The figure shows three views and two pictorial views of one solid part (mm, origin at its lowest corner). Answer the questions. Round coordinates to 2 decimals unless told otherwise and drop trailing zeros. Write each loop counter-clockwise with the first axis right and the second up, starting at its lowest first coordinate (ties: lowest second). Pieces come first, ordered by that corner, then holes. Notation, with made-up numbers: (-16.5, 27.5) -> (-2.5, 27.5) arc R14 ccw to (-2.5, 36.5) -> close; hole circle Ø6 at (58.5, 1.5). An arc over 180 degrees is marked (long way). One line per item, written item: value.
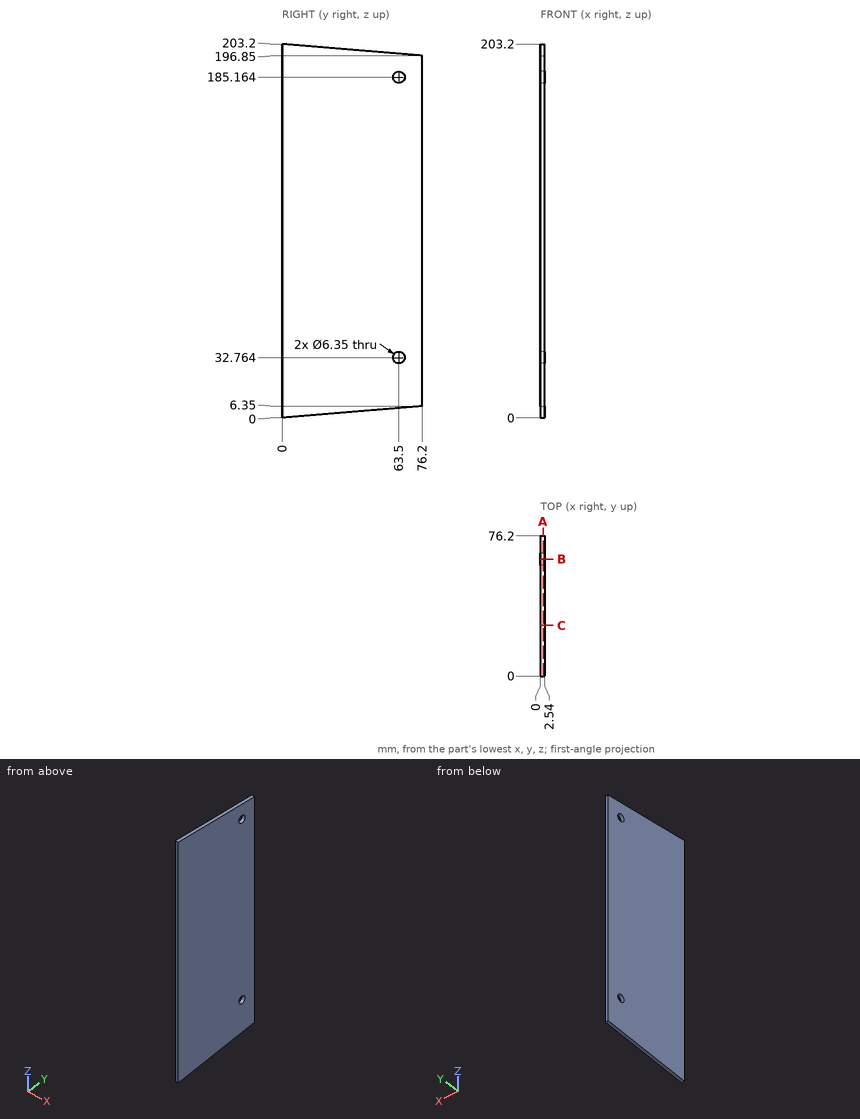
(1) Find section C-C on y = 27.5. Give the vertices of the cut face in (x, z).
Reported:
outline: (0, 2.29) -> (2.54, 2.29) -> (2.54, 200.91) -> (0, 200.91) -> close
(2) Find section B-B on y = 63.5. Give the vertices of the cut face in (x, z), plus the area to 3 significant figures.
Reported:
outline: (0, 5.29) -> (2.54, 5.29) -> (2.54, 29.59) -> (0, 29.59) -> close; (0, 35.94) -> (2.54, 35.94) -> (2.54, 181.99) -> (0, 181.99) -> close; (0, 188.34) -> (2.54, 188.34) -> (2.54, 197.91) -> (0, 197.91) -> close
area: 457 mm2
(3) Consider probe 1 along Z at (x, y) = (1.8, 63.5); probe 2 along Z at (x, y) = (1.2, 65) (1 decimal); probe 3 along Y at (x, z) = (1.75, 184). Determine where each line is inside the solid, lowest interval first.
Reported:
probe 1: z = 5.29 to 29.59, 35.94 to 181.99, 188.34 to 197.91
probe 2: z = 5.4 to 30, 35.6 to 182.4, 188 to 197.8
probe 3: y = 0 to 60.55, 66.45 to 76.2
(4) Find section A-A on x = 1.5. Give the number of separate pieces and of enclosed holes in the cut face, plus the area to 3 significant figures.
Reported:
separate pieces: 1
enclosed holes: 2
area: 14,900 mm2
(5) A flat-ended cylindrical pin translates along its axis: pin 1 Ø1.5 at (x, y) = (2, 31.5) entering from -Z. Find the tip coordinate at first contact, or state that the pin passes through.
Reported:
pin 1: stops at z = 2.56
